from build123d import *

# Parameters (mm, degrees)
SKETCH1_R           = 3.25
BOSS_EXTRUDE1_DEPTH = 50


with BuildPart() as part:
    # Sketch1 → Boss-Extrude1 (new body)
    with BuildSketch(Plane.XY):
        with BuildLine():
            Line((1.5, 0), (38.5, 0))
            ThreePointArc((38.5, 0), (39.560660172, 0.439339828), (40, 1.5))
            Line((40, 1.5), (40, 5.5))
            ThreePointArc((40, 5.5), (39.853553391, 5.853553391), (39.5, 6))
            Line((39.5, 6), (37.5, 6))
            ThreePointArc((37.5, 6), (37.146446609, 5.853553391), (37, 5.5))
            Line((37, 5.5), (37, 2.5))
            ThreePointArc((37, 2.5), (36.853553391, 2.146446609), (36.5, 2))
            Line((36.5, 2), (29.5, 2))
            ThreePointArc((29.5, 2), (29.146446609, 2.146446609), (29, 2.5))
            Line((29, 2.5), (29, 5.5))
            ThreePointArc((29, 5.5), (28.853553391, 5.853553391), (28.5, 6))
            Line((28.5, 6), (26.5, 6))
            ThreePointArc((26.5, 6), (26.146446609, 6.146446609), (26, 6.5))
            Line((26, 6.5), (26, 13.5))
            ThreePointArc((26, 13.5), (26.146446609, 13.853553391), (26.5, 14))
            Line((26.5, 14), (28.5, 14))
            ThreePointArc((28.5, 14), (28.853553391, 14.146446609), (29, 14.5))
            Line((29, 14.5), (29, 17.5))
            ThreePointArc((29, 17.5), (29.146446609, 17.853553391), (29.5, 18))
            Line((29.5, 18), (36.5, 18))
            ThreePointArc((36.5, 18), (36.853553391, 17.853553391), (37, 17.5))
            Line((37, 17.5), (37, 14.5))
            ThreePointArc((37, 14.5), (37.146446609, 14.146446609), (37.5, 14))
            Line((37.5, 14), (39.5, 14))
            ThreePointArc((39.5, 14), (39.853553391, 14.146446609), (40, 14.5))
            Line((40, 14.5), (40, 18.5))
            ThreePointArc((40, 18.5), (39.560660172, 19.560660172), (38.5, 20))
            Line((38.5, 20), (1.5, 20))
            ThreePointArc((1.5, 20), (0.439339828, 19.560660172), (0, 18.5))
            Line((0, 18.5), (0, 14.5))
            ThreePointArc((0, 14.5), (0.146446609, 14.146446609), (0.5, 14))
            Line((0.5, 14), (2.5, 14))
            ThreePointArc((2.5, 14), (2.853553391, 14.146446609), (3, 14.5))
            Line((3, 14.5), (3, 17.5))
            ThreePointArc((3, 17.5), (3.146446609, 17.853553391), (3.5, 18))
            Line((3.5, 18), (10.5, 18))
            ThreePointArc((10.5, 18), (10.853553391, 17.853553391), (11, 17.5))
            Line((11, 17.5), (11, 14.5))
            ThreePointArc((11, 14.5), (11.146446609, 14.146446609), (11.5, 14))
            Line((11.5, 14), (13.5, 14))
            ThreePointArc((13.5, 14), (13.853553391, 13.853553391), (14, 13.5))
            Line((14, 13.5), (14, 6.5))
            ThreePointArc((14, 6.5), (13.853553391, 6.146446609), (13.5, 6))
            Line((13.5, 6), (11.5, 6))
            ThreePointArc((11.5, 6), (11.146446609, 5.853553391), (11, 5.5))
            Line((11, 5.5), (11, 2.5))
            ThreePointArc((11, 2.5), (10.853553391, 2.146446609), (10.5, 2))
            Line((10.5, 2), (3.5, 2))
            ThreePointArc((3.5, 2), (3.146446609, 2.146446609), (3, 2.5))
            Line((3, 2.5), (3, 5.5))
            ThreePointArc((3, 5.5), (2.853553391, 5.853553391), (2.5, 6))
            Line((2.5, 6), (0.5, 6))
            ThreePointArc((0.5, 6), (0.146446609, 5.853553391), (0, 5.5))
            Line((0, 5.5), (0, 1.5))
            ThreePointArc((0, 1.5), (0.439339828, 0.439339828), (1.5, 0))
        make_face()
        with Locations((20, 10)):
            Circle(SKETCH1_R, mode=Mode.SUBTRACT)
    extrude(amount=BOSS_EXTRUDE1_DEPTH)


solid = part.part
Geometry check sheet. Reference: the model listing, model coordinates, mm. A direction names the side the tool comes from. Round coordinates to 2 decimals unless told otherwise and drop trailing zeros. Write each loop counter-clockwise with the first axis right and the second up, starting at its lowest first coordinate (ties: lowest second). Pieces come first, ordered by that corner, then holes.
Item 1: Mould release check, pull along X, two halves, no side actions. Record for faces 4 (the face through (11, 16, 25)), 5 (the face through (0, 17, 25)), 6 (the face through (33, 18, 25)), 7 (the face through (12, 14, 25)): +X half, -X half, draft (parallel to the pull), parting line (faces both ways), or undercut.
Determined:
face 4: undercut
face 5: -X half
face 6: undercut
face 7: draft
Item 2: Section check A-A (y = 10). Record the boundary of the cut face in (x, z), plus the area to 3 significant figures.
Determined:
outline: (14, 0) - (16.75, 0) - (16.75, 50) - (14, 50) - close; (23.25, 0) - (26, 0) - (26, 50) - (23.25, 50) - close
area: 275 mm2
Item 3: Material ranges on line 1 along X through (y, z) = (15.5, 7); line 2 along X through (y, z) = (9.75, 40); line 3 along Y through (x, z) = (20, 34), recorded low to high.
Determined:
line 1: x = 0 to 3, 11 to 29, 37 to 40
line 2: x = 14 to 16.76, 23.24 to 26
line 3: y = 0 to 6.75, 13.25 to 20
Item 4: Section check B-B (x = 4.5). Record the boundary of the cut face in (y, z), plus the area to 3 significant figures.
Determined:
outline: (0, 0) - (2, 0) - (2, 50) - (0, 50) - close; (18, 0) - (20, 0) - (20, 50) - (18, 50) - close
area: 200 mm2
Item 5: Go/stop test with flat-tipped pins: pin 1 Ø5.5 at (y, z) = (10.5, 30.5) entering from -X; pin 2 Ø2 at (y, z) = (11.5, 17.5) entering from +X. Record where each tip stops, or that it passes through.
Determined:
pin 1: stops at x = 14
pin 2: stops at x = 26
Item 6: Access from +Z, -Z, +X, -X, +Y, -Y to the whole of each face (thin tool, end or side, straight path). Record for faces 1 (the face through (29, 16, 25)), 2 (the face through (26, 10, 25)), 3 (the face through (2, 6, 25)).
Determined:
face 1: +Z, -Z
face 2: +Z, -Z, +X
face 3: +Z, -Z, -X
Item 7: Section check C-C (y = 4). Record the boundary of the cut face in (x, z).
Determined:
outline: (0, 0) - (3, 0) - (3, 50) - (0, 50) - close; (11, 0) - (29, 0) - (29, 50) - (11, 50) - close; (37, 0) - (40, 0) - (40, 50) - (37, 50) - close
